```python
from build123d import *

# Parameters (mm, degrees)
F0_W     = 101.5
F0_H     = 38.5
F1_DEPTH = 32
F2_W     = 97.5
F2_H     = 34.5
F3_DEPTH = 29
F5_DEPTH = 38.501
F6_R     = 5
F7_R     = 5
F8_R     = 3


with BuildPart() as f1:
    # F0 (on Top) → F1 (new body)
    with BuildSketch(Plane.XY):
        Rectangle(F0_W, F0_H)
    extrude(amount=F1_DEPTH)

    # F2 (on face) → F3 (cut)
    with BuildSketch(Plane(origin=(0, 0, 0), x_dir=(1, 0, 0), z_dir=(0, 0, -1))):
        Rectangle(F2_W, F2_H)
    extrude(amount=-F3_DEPTH, mode=Mode.SUBTRACT)

    # F4 (on face) → F5 (cut, through all)
    with BuildSketch(Plane.XZ.offset(19.25)):
        with BuildLine():
            Line((-43, 23), (-43, 0))
            Line((-43, 0), (43, 0))
            Line((43, 0), (43, 23))
            ThreePointArc((43, 23), (41.535534, 26.535534), (38, 28))
            Line((38, 28), (-38, 28))
            ThreePointArc((-38, 28), (-41.535534, 26.535534), (-43, 23))
        make_face()
    extrude(amount=-F5_DEPTH, mode=Mode.SUBTRACT)

    # F6
    f6_edges = [f1.edges().sort_by_distance(p)[0] for p in [
        (48.75, 0, 29),
    ]]
    fillet(f6_edges, radius=F6_R)

    # F7
    f7_edges = [f1.edges().sort_by_distance(p)[0] for p in [
        (-48.75, 0, 29),
    ]]
    fillet(f7_edges, radius=F7_R)

    # F8
    f8_edges = [f1.edges().sort_by_distance(p)[0] for p in [
        (50.75, 0, 32),
        (-50.75, 0, 32),
    ]]
    fillet(f8_edges, radius=F8_R)


solid = f1.part
```
Part model, mm, in its own coordinate system. A direction names the side the tool comes from. Round coordinates to 2 decimals unless told otherwise and drop trailing zeros. Write each loop counter-clockwise with the first axis right and the second up, starting at its lowest first coordinate (ties: lowest second). Pieces come first, ordered by that corner, then holes. Notation, with made-up numbers: (28.25, 46.5) -> (33.25, 46.5) arc R27 ccw to (33.25, 70.5) -> close; hole circle Ø7 at (-12.5, 32.25). An arc over 180 degrees is marked (long way). Return JSON: item names as keys, results as strings. Group by question number.
Q1. Saw through at D-D on z = 26. Write the cut outline in (x, y), plus the area to 3 significant figures.
Q2. Pin check, flat tips, straight feed: pin 1 (10.5 mm diameter, centred on x = 6.5, y = -7.5, fed in from -Z); pin 2 (1 mm diameter, centred on x = 11, y = 18, fed in from -Z). Stop position of each tip, or through.
Q3. Probe L1, parallel to X at y = -3, z = 23; L2, parallel to Z at x = 12, y = -13; L3, parallel to Z at x = -28, y = 18.5. List the from-to ranges inside material, lowest first. Write a range as [from, to].
Q4. Which spindle directions (+Z, -Z, +X, -X, +Y, -Y) get a long thin tool onto all of the face, cutting with end or side? Do faces 4 (the cylindrical face through (-41, 18, 27)), 5 (the flat face through (48.75, 0, 12)), 6 (the flat face through (-49, 0, 0)). Say none if no direction does.
Q5. Saw through at C-C on x = 6. Write the cut outline in (y, z).
Q6. Saw through at A-A on z = 16.5. Write the cut outline in (x, y).
Q7. Saw through at B-B on y = -15. Write the cut outline in (x, z).
Q8. Mould opens along X. For faces 1 (the flat face through (49, 0, 0)), 2 (the flat face through (43, 18, 11)), 3 (the flat face through (50.75, 0, 14)) say: pulls with the +X half, pulls with the -X half, needs draft (parallel to the pull), parting line crosses it, or undercut.
Answer:
{
 "1": {"outline": "(-50.75, -19.25) -> (-42, -19.25) -> (-42, -17.25) -> (-48.33, -17.25) -> (-48.33, 17.25) -> (-42, 17.25) -> (-42, 19.25) -> (-50.75, 19.25) -> close; (42, -19.25) -> (50.75, -19.25) -> (50.75, 19.25) -> (42, 19.25) -> (42, 17.25) -> (48.33, 17.25) -> (48.33, -17.25) -> (42, -17.25) -> close", "area": "237 mm2"},
 "2": {"pin 1": "z = 29", "pin 2": "z = 28"},
 "3": {"L1": "[-50.75, -48.75], [48.75, 50.75]", "L2": "[29, 32]", "L3": "[28, 32]"},
 "4": {"face 4": "-Z, +Y, -Y", "face 5": "-Z", "face 6": "-Z, +X, -X, +Y, -Y"},
 "5": {"outline": "(-19.25, 28) -> (-17.25, 28) -> (-17.25, 29) -> (17.25, 29) -> (17.25, 28) -> (19.25, 28) -> (19.25, 32) -> (-19.25, 32) -> close"},
 "6": {"outline": "(-50.75, -19.25) -> (-43, -19.25) -> (-43, -17.25) -> (-48.75, -17.25) -> (-48.75, 17.25) -> (-43, 17.25) -> (-43, 19.25) -> (-50.75, 19.25) -> close; (43, -19.25) -> (50.75, -19.25) -> (50.75, 19.25) -> (43, 19.25) -> (43, 17.25) -> (48.75, 17.25) -> (48.75, -17.25) -> (43, -17.25) -> close"},
 "7": {"outline": "(-50.75, 0) -> (-48.75, 0) -> (-48.75, 24) arc R5 cw to (-43.75, 29) -> (43.75, 29) arc R5 cw to (48.75, 24) -> (48.75, 0) -> (50.75, 0) -> (50.75, 29) arc R3 ccw to (47.75, 32) -> (-47.75, 32) arc R3 ccw to (-50.75, 29) -> close"},
 "8": {"face 1": "needs draft", "face 2": "undercut", "face 3": "pulls with the +X half"}
}
